CAD build for the part. Positions are in the model's coordinates, mm. Round coordinates to 2 decimals unless told otherwise and drop trailing zeros. Write each loop counter-clockwise with the first axis right and the second up, starting at its lowest first coordinate (ties: lowest second). Pieces come first, ordered by that corner, then holes. Notation, with made-up numbers: (37, 42) - (67, 42) arc R14 cw to (67, 54) - close; hole circle Ø5 at (15, 58.25). An arc over 180 degrees is marked (long way). Use one line per item in the form item = value. Start each with the question number.
Item 1: Pin check, flat tip, straight feed: pin 1 (4 mm diameter, centred on x = -2.9, y = -0.1, fed in from -Z). Stop position of the tip, or through.
Item 2: Band-saw the part on B-B, the plane z = 1.3. List the corners of the cut face in (x, y).
Item 3: Band-saw the part on A-A, the plane x = -2.9. List the corners of the cut face in (y, z), and give its area (3 significant figures).
Item 4: Drill centre lines: L1, parallel to X at y = 0, z = 1.4; L2, parallel to Y at x = 30, z = 2; L3, parallel to Y at x = -2.9, z = 0.85. Where is each one in solid material? Low to high.
Autodesk Inventor part; units mm, degrees
ref_plane "YZ Plane" through (0, 0, 0) normal (1, 0, 0) x (0, 1, 0)
ref_plane "XZ Plane" through (0, 0, 0) normal (0, 1, 0) x (-1, 0, 0)
ref_plane "XY Plane" through (0, 0, 0) normal (0, 0, 1) x (1, 0, 0)
sketch "Sketch1" plane through (0, 0, 0) normal (0, 0, 1) x (1, 0, 0)
  line L0 (-30, 10) -> (30, 10)
  line L1 (35, 5) -> (35, -5)
  line L2 (30, -10) -> (-30, -10)
  line L3 (-35, -5) -> (-35, 5)
  line L4 (-50.4497, 0) -> (50.4497, 0)
  line L5 (0, -15.4497) -> (0, 15.4497)
  arc A0 (-30, 10) -> (-35, 5) centre (-30, 5) ccw
  arc A1 (-35, -5) -> (-30, -10) centre (-30, -5) ccw
  arc A2 (30, -10) -> (35, -5) centre (30, -5) ccw
  arc A3 (35, 5) -> (30, 10) centre (30, 5) ccw
  circle A4 centre (-30, 0) radius 1.5
  circle A5 centre (30, 0) radius 1.5
  circle A6 centre (-2.9, -0.1) radius 1.5
  point P0 (0, 0)
  point P1 (-35, 10)
  point P2 (35, -10)
  point P3 (35, 10)
  point P4 (-35, -10)
  dimension "d2" = 70
  dimension "d3" = 35
  dimension "d4" = 20
  dimension "d5" = 10
  dimension "d6" = 5
  dimension "d9" = 3
  dimension "d10" = 3
extrude "Extrusion2" add sketch "Sketch1" along normal blind 2.8 contours L0 L5 L4 A6 A4 L3 A0 | L0 A3 L1 L4 A5 L5 | L5 L2 A1 L3 L4 A4 A6 | L4 A5 L1 A2 L2 L5
equation "\"d3\" = 0.5 * d2"
equation "\"d5\" = 0.5 * d4"
properties part number "Acrylic_YawServoSupport_4"
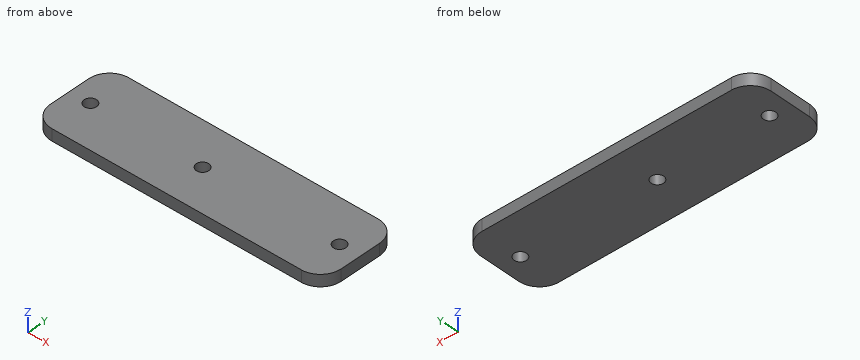
Determined:
q1.pin_1 = 0
q2.outline = (-35, -5) arc R5 ccw to (-30, -10) - (30, -10) arc R5 ccw to (35, -5) - (35, 5) arc R5 ccw to (30, 10) - (-30, 10) arc R5 ccw to (-35, 5) - close; hole circle Ø3 at (-30, 0); hole circle Ø3 at (-2.9, -0.1); hole circle Ø3 at (30, 0)
q3.outline = (-10, 0) - (-1.6, 0) - (-1.6, 2.8) - (-10, 2.8) - close; (1.4, 0) - (10, 0) - (10, 2.8) - (1.4, 2.8) - close
q3.area = 47.6 mm²
q4.L1 = -35 to -31.5, -28.5 to -4.4, -1.4 to 28.5, 31.5 to 35
q4.L2 = -10 to -1.5, 1.5 to 10
q4.L3 = -10 to -1.6, 1.4 to 10
